Part print with two shaded views. Sizes in mm from the minimum x, y, z corner. Round coordinates to 2 decimals unless told otherwise and drop trailing zeros. Order: outer loops, then holes, each group sorted by start corner. A loop starts at its lowest first (then second) coordinate and runs counter-clockwise, first axis right, second up. Notation, with made-up numbers: M 62.25,19.25 L 94.25,19.25 A29 cw 94.25,49.25 Z; hole C -38,-17 d11. An arc over 180 degrees is marked long. Answer as a JSON object with one key per item and string values.
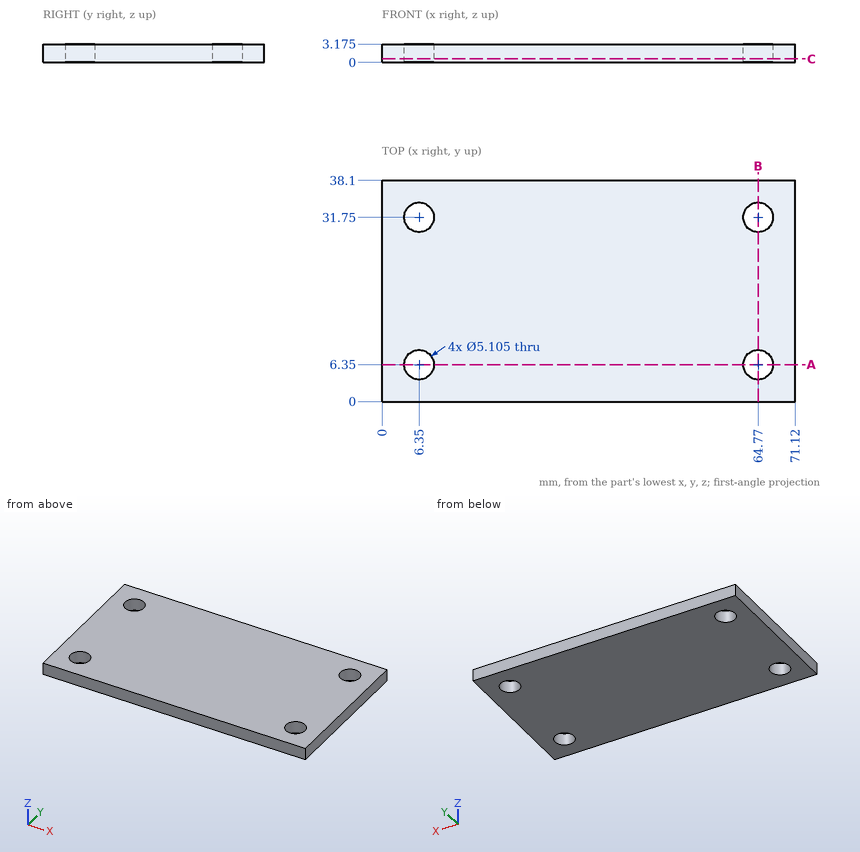
Item 1: Wall check: line 1 along Y through (x, z) = (64.77, 0.7); line 2 along X through (y, z) = (33, 0.2) (1 decimal); line 3 along X through (y, z) = (34, 3) (1 decimal). Give the ranges that are in metal, low to high. Write a range as [from, to].
Worked answers:
{"line 1": "y = [0, 3.8], [8.9, 29.2], [34.3, 38.1]", "line 2": "x = [0, 4.1], [8.6, 62.5], [67, 71.1]", "line 3": "x = [0, 5.1], [7.6, 63.6], [66, 71.1]"}
Item 2: Saw through at A-A on y = 6.35. List the corners of the cut face in (x, z) (1 decimal), and give its area (3 significant figures).
Worked answers:
{"outline": "M 0,0 L 3.8,0 L 3.8,3.2 L 0,3.2 Z; M 8.9,0 L 62.2,0 L 62.2,3.2 L 8.9,3.2 Z; M 67.3,0 L 71.1,0 L 71.1,3.2 L 67.3,3.2 Z", "area": "193 mm2"}
Item 3: Saw through at B-B on x = 64.77. List the corners of the cut face in (y, z) (1 decimal).
Worked answers:
{"outline": "M 0,0 L 3.8,0 L 3.8,3.2 L 0,3.2 Z; M 8.9,0 L 29.2,0 L 29.2,3.2 L 8.9,3.2 Z; M 34.3,0 L 38.1,0 L 38.1,3.2 L 34.3,3.2 Z"}
Item 4: Saw through at C-C on z = 0.6. State how many separate pieces and enclosed holes the cut face has, and give its area (3 significant figures).
Worked answers:
{"separate pieces": "1", "enclosed holes": "4", "area": "2,630 mm2"}
